Part model, mm, in its own coordinate system. A direction names the side the tool comes from. Coordinates: 2 decimals unless noted, no trailing zeros. Loops run counter-clockwise (first coordinate to the right, second up) from the corner with the lowest first, then second, coordinate; pieces in that order, holes last. Notation, with made-up numbers: (-23, 4) - (0, 4) arc R13 cw to (0, 22) - close; hole circle Ø1 at (47.5, 61). An arc over 180 degrees is marked (long way). Use a Markdown table: item, result. Add a question column.
1) Probe probe 1 along Y at (x, z) = (2, -2.25); probe 2 along X at (y, z) = (14, 8.5); probe 3 along X at (y, z) = (9, 11.25). List the from-to ranges inside material, lowest first. Write a range as [from, to].
2) Tool access for faces 4 (the face through (2, -5, -11)), 5 (the face through (9.294, 22.042, -4.419)), 6 (the face through (-9.302, -2.465, 0.327)), 7 (the face through (-1.334, -2.465, -11.61)): list every direction of +Z, -Z, +X, -X, +Y, -Y with a clear straight run to the whole face (end or side of a thin tool).
3) Pull direction Y, two halves, no side cores. Call faces 1 (the face through (0, 0, 0)), 2 (the face through (11.367, -2.465, -2.416)), 3 (the face through (-1.502, 24.042, -11.443)): +Y half, -Y half, draft (parallel to the pull), parting line (faces both ways), or undercut.
4) Band-saw the part on C-C (y = 9.5). Give the cut face in (x, z).
5) Drop flat-ended pins along their axis: P1, Ø12, axis at y = 33.5, z = 8, coming from the -X side; P2, Ø5, axis at y = -2.5, z = 12.5, coming from the -X side; P3, Ø1.5, axis at y = 23.5, z = 12.5, coming from the -X side; P4, Ø12, axis at x = -9, y = 37, coming from the -Z side. Give the stop position or say it passes through.
6) Band-saw the part on A-A (z = 0). Give the cut face in (x, y), plus the area to 3 significant figures.
7) Band-saw the part on B-B (y = 23). Give the number of separate pieces and of enclosed holes in the cut face, plus the area to 3 significant figures.
from build123d import *

# Parameters (mm, degrees)
SKETCH1_R             = 14
BOSS_EXTRUDE1_DEPTH   = 25
CHAMFER1_SIZE         = 6
CHAMFER1_SIZE2        = 2.926395531
CUT_EXTRUDE1_DEPTH    = 6
CIRPATTERN1_COUNT     = 10
SKETCH3_R             = 13.212713
BOSS_EXTRUDE2_DEPTH   = 4
CHAMFER2_SIZE         = 1.5
CHAMFER2_SIZE2        = 1.787630389
CHAMFER2_PART_2_SIZE  = 1.5
CHAMFER2_PART_2_SIZE2 = 1.787630389
SKETCH4_R             = 2
BOSS_EXTRUDE3_DEPTH   = 24
BOSS_EXTRUDE4_DEPTH   = 5
CIRPATTERN2_COUNT     = 7
CIRPATTERN2_ANGLE     = 306


with BuildPart() as part:
    # Sketch1 → Boss-Extrude1 (new body)
    with BuildSketch(Plane(origin=(0, 0, 0), x_dir=(1, 0, 0), z_dir=(0, 1, 0))):
        Circle(SKETCH1_R)
    extrude(amount=BOSS_EXTRUDE1_DEPTH)

    # Chamfer1
    chamfer1_edges = [part.edges().sort_by_distance(p)[0] for p in [
        (-14, 25, 0),
    ]]
    chamfer1_side = [part.faces().sort_by_distance(p)[0] for p in [
        (-14, 12.5, 0),
    ]]
    chamfer(chamfer1_edges, length=CHAMFER1_SIZE, length2=CHAMFER1_SIZE2, reference=chamfer1_side[0])

    # Sketch2 → Cut-Extrude1 (cut)
    with BuildSketch(Plane(origin=(0, 25, 0), x_dir=(1, 0, 0), z_dir=(0, 1, 0))):
        with BuildLine():
            Line((0, 10.291206374), (0, 13.212713))
            ThreePointArc((0, 13.212713), (2.447017171, 12.98414001), (4.80937012, 12.306329423))
            Line((4.80937012, 12.306329423), (3.745954402, 9.585236265))
            ThreePointArc((3.745954402, 9.585236265), (-1.905949119, -10.113173913), (0, 10.291206374))
        make_face()
    cut_extrude1 = extrude(amount=-CUT_EXTRUDE1_DEPTH, mode=Mode.SUBTRACT)

    # CirPattern1: Cut-Extrude1 ×10 about axis
    cirpattern1_axis = Axis((0, 0, 0), (0, 1, 0))
    for i in range(1, CIRPATTERN1_COUNT):
        add(cut_extrude1.rotate(cirpattern1_axis, i * 360 / CIRPATTERN1_COUNT), mode=Mode.SUBTRACT)

    # Sketch3 → Boss-Extrude2 (add)
    with BuildSketch(Plane(origin=(0, 25, 0), x_dir=(1, 0, 0), z_dir=(0, 1, 0))):
        Circle(SKETCH3_R)
    extrude(amount=BOSS_EXTRUDE2_DEPTH)

    # Chamfer2
    chamfer2_edges = [part.edges().sort_by_distance(p)[0] for p in [
        (-13.212713, 25, 0),
    ]]
    chamfer2_side = [part.faces().sort_by_distance(p)[0] for p in [
        (0, 25, 0),
    ]]
    chamfer(chamfer2_edges, length=CHAMFER2_SIZE, length2=CHAMFER2_SIZE2, reference=chamfer2_side[0])

    # Chamfer2 part 2
    chamfer2_part_2_edges = [part.edges().sort_by_distance(p)[0] for p in [
        (-13.212713, 29, 0),
    ]]
    chamfer2_part_2_side = [part.faces().sort_by_distance(p)[0] for p in [
        (-13.212713, 27, 0),
    ]]
    chamfer(chamfer2_part_2_edges, length=CHAMFER2_PART_2_SIZE, length2=CHAMFER2_PART_2_SIZE2, reference=chamfer2_part_2_side[0])

    # Sketch4 → Boss-Extrude3 (add)
    with BuildSketch(Plane(origin=(0, 19, 0), x_dir=(1, 0, 0), z_dir=(0, 1, 0))):
        Circle(SKETCH4_R)
    extrude(amount=BOSS_EXTRUDE3_DEPTH)

    # Sketch5 → Boss-Extrude4 (add)
    with BuildSketch(Plane.XZ):
        with BuildLine():
            Line((0, 9.308060502), (0, 14))
            ThreePointArc((0, 14), (4.041174246, 13.404063217), (7.738307866, 11.666987245))
            Line((7.738307866, 11.666987245), (5.1449027, 7.756930225))
            ThreePointArc((5.1449027, 7.756930225), (2.686821027, 8.911845099), (0, 9.308060502))
        make_face()
    boss_extrude4 = extrude(amount=BOSS_EXTRUDE4_DEPTH)

    # CirPattern2: Boss-Extrude4 ×7 about axis
    cirpattern2_axis = Axis((0, 0, 0), (0, 1, 0))
    for i in range(1, CIRPATTERN2_COUNT):
        add(boss_extrude4.rotate(cirpattern2_axis, i * CIRPATTERN2_ANGLE / (CIRPATTERN2_COUNT - 1)))


solid = part.part
Answer block:
| question | item | result |
|---|---|---|
| 1 | probe 1 | [0, 19], [25, 29] |
| 1 | probe 2 | [-11.12, 11.12] |
| 1 | probe 3 | [-8.33, 8.33] |
| 2 | face 4 | +Z, -Z, +X, -X, -Y |
| 2 | face 5 | none |
| 2 | face 6 | -Y |
| 2 | face 7 | +Z, -Y |
| 3 | face 1 | -Y half |
| 3 | face 2 | draft |
| 3 | face 3 | undercut |
| 4 | outline | circle Ø28 at (0, 0) |
| 5 | P1 | x = -11.32 |
| 5 | P2 | x = -9.8 |
| 5 | P3 | x = 0 |
| 5 | P4 | through |
| 6 | outline | (-14, -5) - (-9.31, -5) - (-9.31, 0) - (14, 0) - (14, 19) - (13.21, 20.61) - (13.21, 19) - (2, 19) - (2, 25) - (11.71, 25) - (13.21, 26.79) - (13.21, 27.5) - (11.43, 29) - (2, 29) - (2, 43) - (-2, 43) - (-2, 29) - (-11.43, 29) - (-13.21, 27.5) - (-13.21, 26.79) - (-11.71, 25) - (-2, 25) - (-2, 19) - (-13.21, 19) - (-13.21, 20.61) - (-14, 19) - close |
| 6 | area | 737 mm2 |
| 7 | separate pieces | 11 |
| 7 | enclosed holes | 0 |
| 7 | area | 62.8 mm2 |
